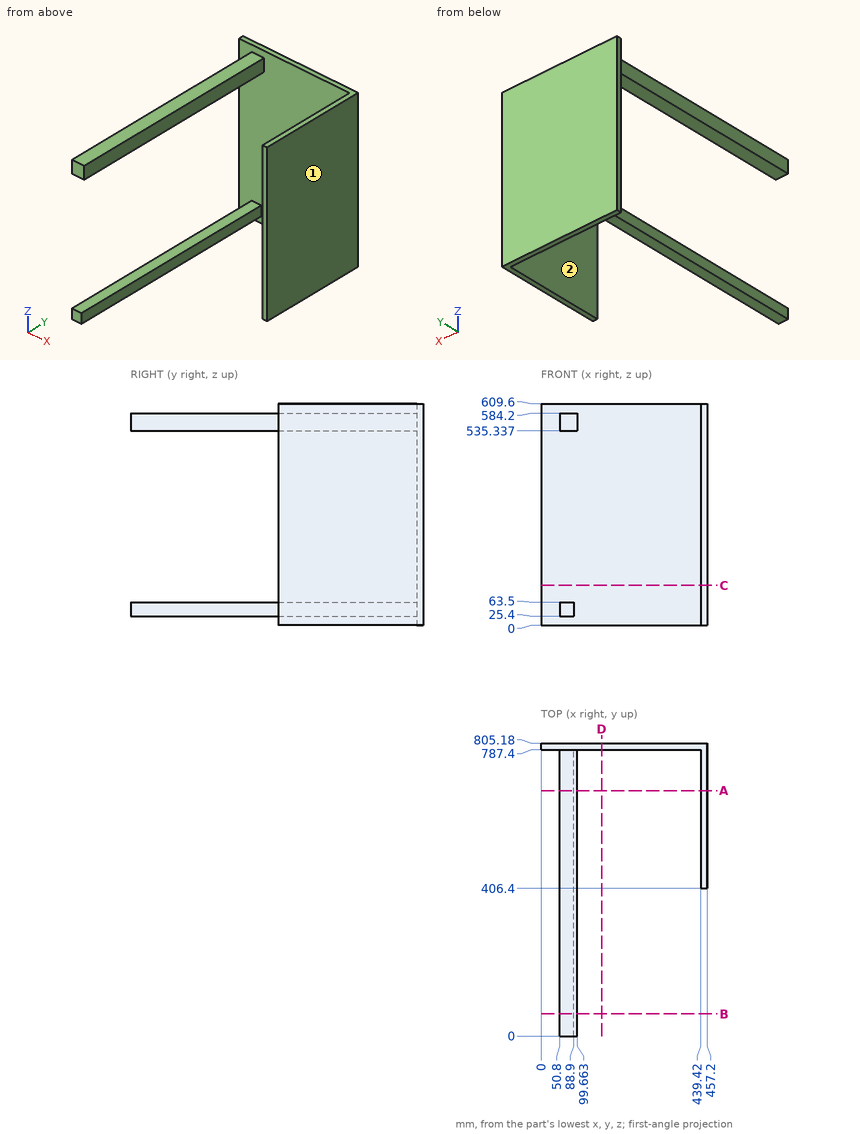
The figure shows three views and two pictorial views of one solid part (mm, origin at its lowest corner). Answer the questions. A direction names the side the tool comes from. Give positions to 0.01 mm unless a question says otherwise; leave off trailing zeros. Write each loop counter-clockwise with the first axis right and the second up, starting at its lowest first coordinate (ties: lowest second). Pieces come first, ordered by that corner, then holes.
Q1. A tool of negligible diameter and unlimited length cuts with its end or side. For the marked faces 1 and 2, from which of +Z, -Z, +X, -X, +Y, -Y can it reach the whole face along a straight path? Write none if from no direction.
Answer:
face 1: +Z, -Z, +X, +Y, -Y
face 2: +Z, -Z, -Y
Q2. The part is cut by section B-B on y = 61. Give the vertices of the cut face in (x, z), and give its area (3 significant figures).
Answer:
outline: (50.8, 25.4) - (88.9, 25.4) - (88.9, 63.5) - (50.8, 63.5) - close; (50.8, 535.34) - (99.66, 535.34) - (99.66, 584.2) - (50.8, 584.2) - close
area: 3,840 mm2
Q3. Given pin 1 (11.5 mm diameter, centred on y = 296.5, z = 35.5, fed in from -X); pin 2 (5.5 mm diameter, centred on x = 448.5, z = 272.5, fed in from -Y); pin 3 (14.5 mm diameter, centred on x = 65.5, y = 212.5, fed in from -Z), each flat-ended and moving along its own axis, determine where each tip first touches the part or whether it passes through.
Answer:
pin 1: stops at x = 50.8
pin 2: stops at y = 406.4
pin 3: stops at z = 25.4
Q4. The part is cut by section D-D on x = 166. Give the vertices of the cut face in (y, z).
Answer:
outline: (787.4, 0) - (805.18, 0) - (805.18, 609.6) - (787.4, 609.6) - close
Q5. The part is cut by section A-A on y = 675.5. Give the vertices of the cut face in (x, z), and give its area (3 significant figures).
Answer:
outline: (50.8, 25.4) - (88.9, 25.4) - (88.9, 63.5) - (50.8, 63.5) - close; (50.8, 535.34) - (99.66, 535.34) - (99.66, 584.2) - (50.8, 584.2) - close; (439.42, 0) - (457.2, 0) - (457.2, 609.6) - (439.42, 609.6) - close
area: 14,700 mm2
Q6. The part is cut by section C-C on z = 110.5. Give the vertices of the cut face in (x, y).
Answer:
outline: (0, 787.4) - (439.42, 787.4) - (439.42, 406.4) - (457.2, 406.4) - (457.2, 805.18) - (0, 805.18) - close
Q7. Straight lines are drawn through the part: L1, parallel to X at y = 669.5, z = 573.5; L2, parallel to Y at x = 291.5, z = 383.5; L3, parallel to X at y = 374, z = 566. For each, find the intervals that lie inside material, in ascending order.
Answer:
L1: x = 50.8 to 99.66, 439.42 to 457.2
L2: y = 787.4 to 805.18
L3: x = 50.8 to 99.66
